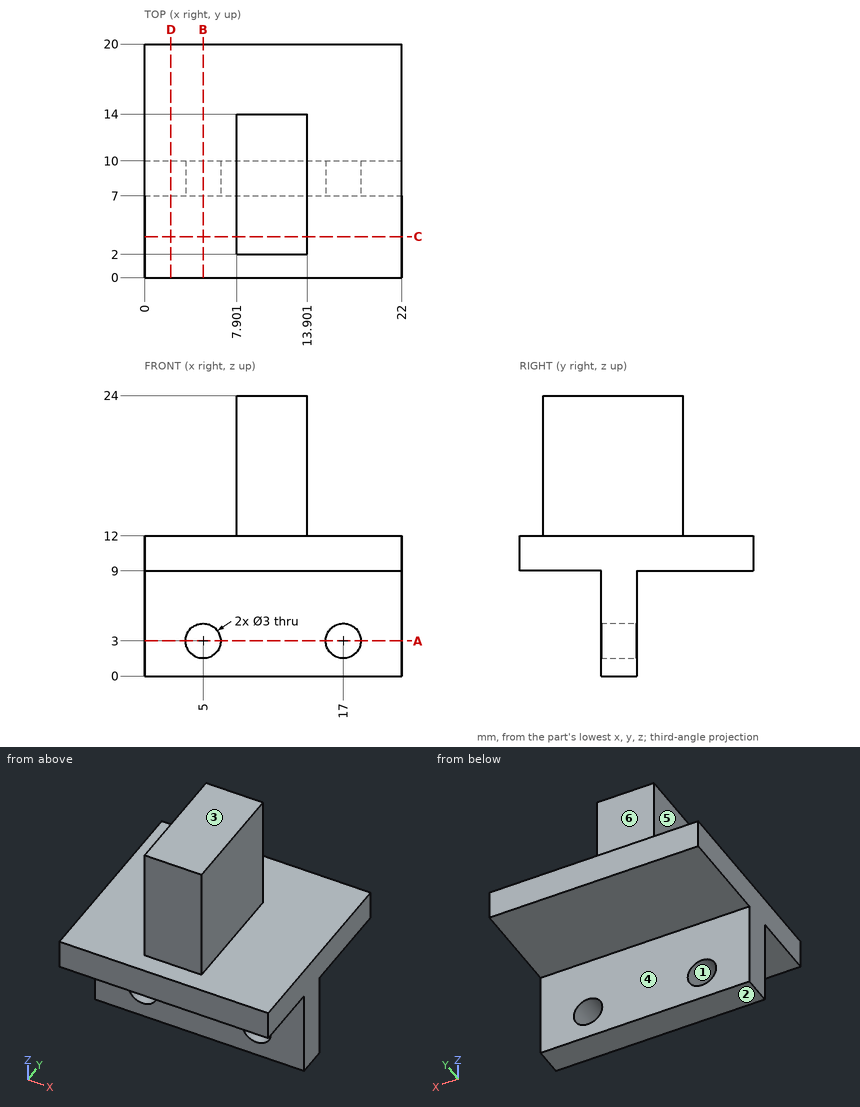
Can you work these out from the drawing? Everything is in mm from the part's minimum corner. A direction names the side the tool comes from. Coordinates: 2 decimals unless noted, no trailing zeros. Loops run counter-clockwise (first coordinate to the right, second up) from the corner with the lowest first, then second, coordinate; pieces in that order, holes last. Notation, with made-up numbers: (-9.5, -39.75) - (18.5, -39.75) arc R11 ccw to (18.5, -29.75) - close; hole circle Ø2 at (-6.75, 75.5). An arc over 180 degrees is marked (long way). Use a Markdown table: item, result.
Item 1: For the marked faces 4, 5 and 6, which set-ups out of +Z, -Z, +X, -X, +Y, -Y let a thin tool reach every point of the face, with its end or its side?
Numbers:
| item | result |
|---|---|
| face 4 | -Z, +X, -X, +Y |
| face 5 | +Z, -X, +Y, -Y |
| face 6 | +Z, +X, -X, +Y |
Item 2: I want a section at C-C on y = 3.5. Please give me the cut outline in (x, z).
Numbers:
| item | result |
|---|---|
| outline | (0, 9) - (22, 9) - (22, 12) - (13.9, 12) - (13.9, 24) - (7.9, 24) - (7.9, 12) - (0, 12) - close |
Item 3: I want a section at A-A on z = 3. Please give me the cut outline in (x, y).
Numbers:
| item | result |
|---|---|
| outline | (0, 7) - (3.5, 7) - (3.5, 10) - (0, 10) - close; (6.5, 7) - (15.5, 7) - (15.5, 10) - (6.5, 10) - close; (18.5, 7) - (22, 7) - (22, 10) - (18.5, 10) - close |
Item 4: I want a section at D-D on x = 2.25. Please give me the cut outline in (y, z).
Numbers:
| item | result |
|---|---|
| outline | (0, 9) - (7, 9) - (7, 0) - (10, 0) - (10, 9) - (20, 9) - (20, 12) - (0, 12) - close |
Item 5: If I drill on probe 1 along X at (y, z) = (8.55, 3); probe 2 along Z at (x, y) = (17, 7.75); probe 3 along Z at (x, y) = (2.25, 17.5), over which ranges is the centre line in solid material (lowest first)? Write a range as from..to.
Numbers:
| item | result |
|---|---|
| probe 1 | x = 0..3.5, 6.5..15.5, 18.5..22 |
| probe 2 | z = 0..1.5, 4.5..12 |
| probe 3 | z = 9..12 |
Item 6: Will these pins go through, and if not, where does the flat tip stop? pin 1 (5.5 mm diameter, centred on x = 11, y = 2.5, fed in from -Z); pin 2 (5 mm diameter, centred on x = 5, z = 3, fed in from -Y); pin 3 (3 mm diameter, centred on y = 15, z = 7, fed in from +X); pin 4 (1.8 mm diameter, centred on x = 9.5, z = 19, fed in from +Y).
Numbers:
| item | result |
|---|---|
| pin 1 | stops at z = 9 |
| pin 2 | stops at y = 7 |
| pin 3 | passes through |
| pin 4 | stops at y = 14 |
Item 7: I want a section at B-B on x = 5. Please give me the cut outline in (y, z).
Numbers:
| item | result |
|---|---|
| outline | (0, 9) - (7, 9) - (7, 4.5) - (10, 4.5) - (10, 9) - (20, 9) - (20, 12) - (0, 12) - close; (7, 0) - (10, 0) - (10, 1.5) - (7, 1.5) - close |
Item 8: We'd pull the mould along Z, two halves only. Please class the marked faces 1, 2 and 3: released by +Z, released by -Z, zero draft, split by the parting line, or undercut.
Numbers:
| item | result |
|---|---|
| face 1 | undercut |
| face 2 | released by -Z |
| face 3 | released by +Z |
